Geometry: see drawing. Coordinates: mm, zero at the bounding-box minimum. A direction names the side the tool comes from. Give positions to 0.01 mm unless a question says otherwise; leave off trailing zeros. Write each loop counter-clockwise with the first axis right and the second up, starting at its lowest first coordinate (ties: lowest second). Pieces come first, ordered by that corner, then holes. Notation, with made-up numbers: (72, 39) -> (82, 39) arc R22 ccw to (82, 45) -> close; hole circle Ø2 at (-33.75, -23.5). An arc over 180 degrees is marked (long way). Use CSV: the item, a comma, the result in double quotes. Start each with the question number.
1) Material intervals for line 1 (X direction, y = 12.35, z = 87); line 2 (X direction, y = 13.3, z = 5); line 3 (Z direction, x = 79, y = 11.4), sorted ascending. Write a range as [from, to].
2) Section B-B (y = 6). Output: boundary loops of the cut face in (x, z), plus the area to 4 significant figures.
3) Contact query for flat-ended pins moving along their axis: P1, Ø2.5, axis at x = 43, y = 6, coming from the +Z side; P2, Ø2, axis at x = 49.5, z = 37, coming from the -Y side; P3, Ø1.5, axis at y = 9, z = 21, coming from the +X side; P4, Ø5, axis at x = 44, y = 6, coming from the -Z side. Output: stop coordinate, or through.
4) Section C-C (x = 79). Output: boundary loops of the cut face in (y, z).
5) Section A-A (z = 60). Output: boundary loops of the cut face in (x, y).
6) Section D-D (x = 42). Output: boundary loops of the cut face in (y, z).
7) Set-up query: the marked faces 1 and 2. Return all of +Z, -Z, +X, -X, +Y, -Y with unobstructed straight access to the full face (end or side cutting, diameter ignored); none if empty.
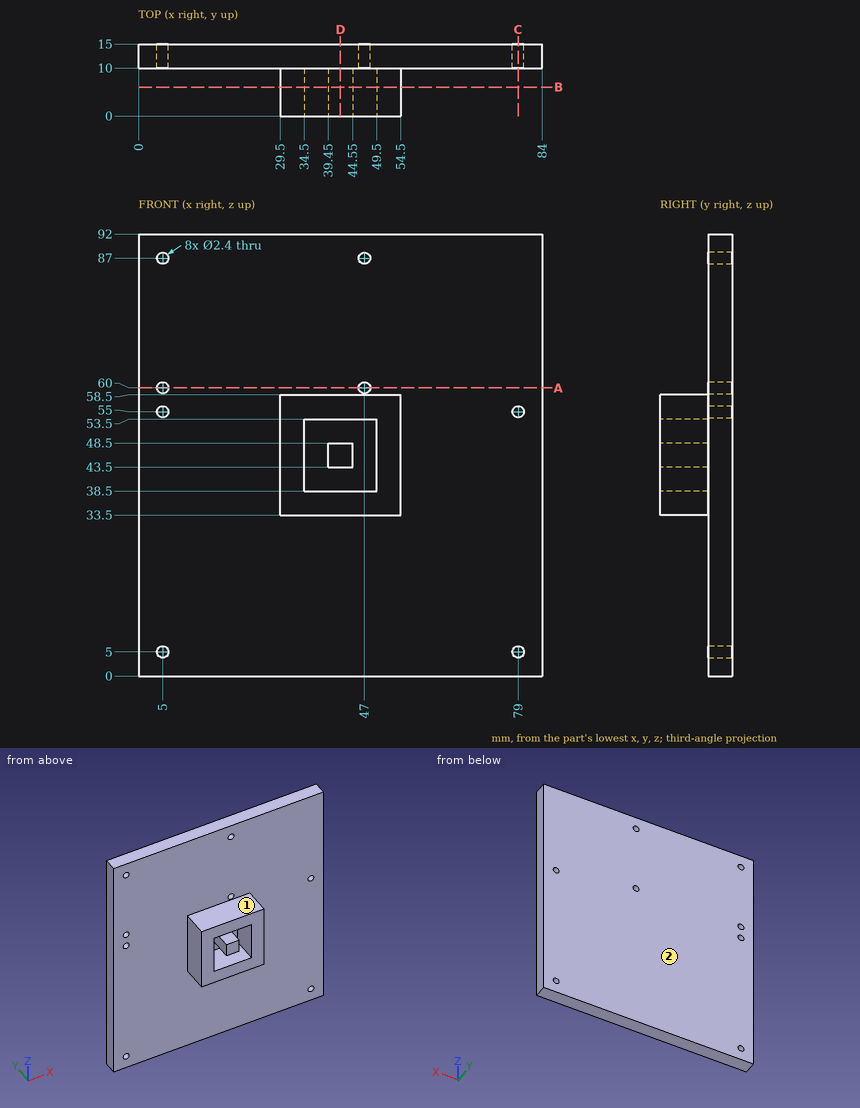
Answers follow:
1,line 1,"x = [0, 3.8], [6.2, 45.8], [48.2, 84]"
1,line 2,"x = [0, 3.8], [6.2, 77.8], [80.2, 84]"
1,line 3,"z = [0, 3.8], [6.2, 53.8], [56.2, 92]"
2,outline,"(29.5, 33.5) -> (54.5, 33.5) -> (54.5, 58.5) -> (29.5, 58.5) -> close; (39.45, 43.5) -> (44.55, 43.5) -> (44.55, 48.5) -> (39.45, 48.5) -> close; hole (34.5, 38.5) -> (49.5, 38.5) -> (49.5, 53.5) -> (34.5, 53.5) -> close"
2,area,"425.5 mm^2"
3,P1,"stops at z = 58.5"
3,P2,"stops at y = 0"
3,P3,"passes through"
3,P4,"stops at z = 33.5"
4,outline,"(10, 0) -> (15, 0) -> (15, 3.8) -> (10, 3.8) -> close; (10, 6.2) -> (15, 6.2) -> (15, 53.8) -> (10, 53.8) -> close; (10, 56.2) -> (15, 56.2) -> (15, 92) -> (10, 92) -> close"
5,outline,"(0, 10) -> (3.8, 10) -> (3.8, 15) -> (0, 15) -> close; (6.2, 10) -> (45.8, 10) -> (45.8, 15) -> (6.2, 15) -> close; (48.2, 10) -> (84, 10) -> (84, 15) -> (48.2, 15) -> close"
6,outline,"(0, 33.5) -> (10, 33.5) -> (10, 0) -> (15, 0) -> (15, 92) -> (10, 92) -> (10, 58.5) -> (0, 58.5) -> (0, 53.5) -> (10, 53.5) -> (10, 48.5) -> (0, 48.5) -> (0, 43.5) -> (10, 43.5) -> (10, 38.5) -> (0, 38.5) -> close"
7,face 1,"+Z, +X, -X, -Y"
7,face 2,"+Z, -Z, +X, -X, +Y"
